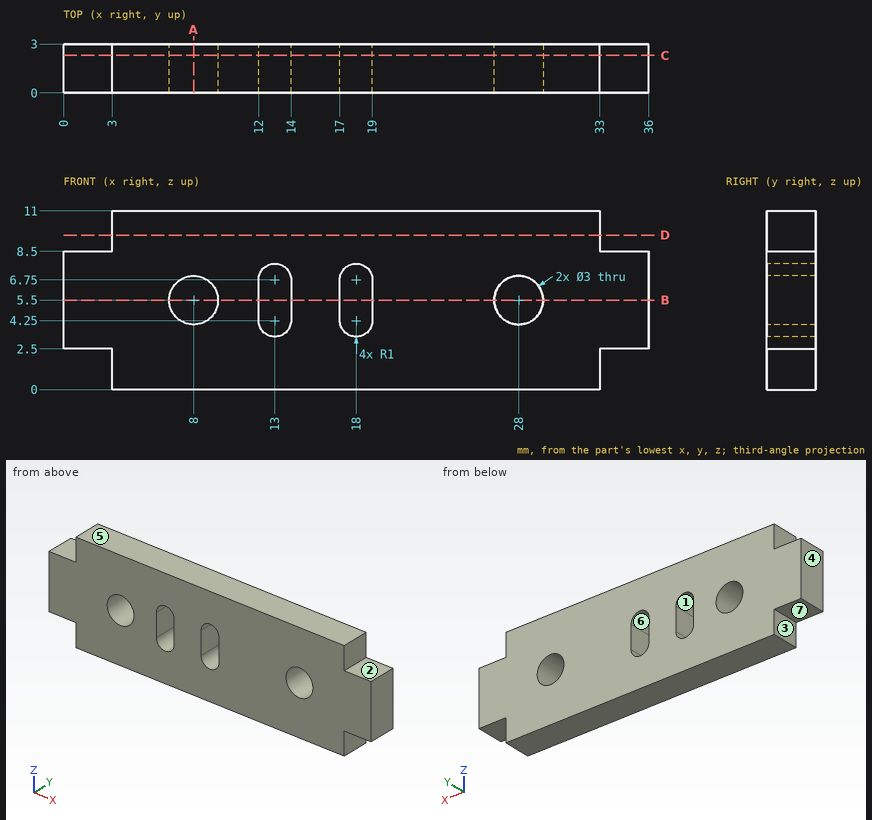
The drawing under review shows one solid part. Ordinate dimensions are in mm from its lowest x, y, z. A direction names the side the tool comes from. Round coordinates to 2 decimals unless told otherwise and drop trailing zeros. Write each loop counter-clockwise with the first axis right and the second up, starting at its lowest first coordinate (ties: lowest second). Pieces come first, ordered by that corner, then holes. Notation, with made-up numbers: (-1, 46) - (40, 46) arc R33 cw to (40, 75) - close; hole circle Ø3 at (5, 13.25). An arc over 180 degrees is marked (long way). Put each result on its own line as item: value.
Q1. We need section D-D (z = 9.5). Give the boundary of the cut face in (x, y), and give its area (3 significant figures).
Solved:
outline: (3, 0) - (33, 0) - (33, 3) - (3, 3) - close
area: 90.0 mm2
Q2. Wall thickness on probe 1 along Z at (x, y) = (28, 1.25); probe 2 along X at (y, z) = (2.7, 4.5); probe 3 along X at (y, z) = (2.8, 5): over which ranges is each line inside the solid? List them lowest first.
Solved:
probe 1: z = 0 to 4, 7 to 11
probe 2: x = 0 to 6.88, 9.12 to 12, 14 to 17, 19 to 26.88, 29.12 to 36
probe 3: x = 0 to 6.59, 9.41 to 12, 14 to 17, 19 to 26.59, 29.41 to 36
Q3. We need section B-B (z = 5.5). Give the boundary of the cut face in (x, y), and give its area (3 significant figures).
Solved:
outline: (0, 0) - (6.5, 0) - (6.5, 3) - (0, 3) - close; (9.5, 0) - (12, 0) - (12, 3) - (9.5, 3) - close; (14, 0) - (17, 0) - (17, 3) - (14, 3) - close; (19, 0) - (26.5, 0) - (26.5, 3) - (19, 3) - close; (29.5, 0) - (36, 0) - (36, 3) - (29.5, 3) - close
area: 78.0 mm2
Q4. Machinability: for the marked faces 1, 2 and 3, which of the approach directions +Z, -Z, +X, -X, +Y, -Y give a long, thin tool a straight path to every point of the face, cutting with its end or side? Answer none if there is none.
Solved:
face 1: +Y, -Y
face 2: +Z, +X, +Y, -Y
face 3: -Z, -X, +Y, -Y
Q5. Mouldability with a two-part tool opening along Z and no side actions: class the marked faces 4, 5, 6 and 7 as released by +Z, released by -Z, zero draft, split by the parting line, or undercut.
Solved:
face 4: zero draft
face 5: released by +Z
face 6: undercut
face 7: released by -Z
Q6. Insertion check: pin 1 Ø0.9 at (x, y) = (35, 1) entering from +Z; pin 2 Ø1.2 at (y, z) = (2, 9.5) entering from -X; pin 3 Ø1.5 at (x, y) = (2, 1) entering from -Z. Each pin has a flat end and moves straight along its axis. Give the tip position at first contact, or say it passes through.
Solved:
pin 1: stops at z = 8.5
pin 2: stops at x = 3
pin 3: stops at z = 2.5
Q7. We need section A-A (x = 8). Give the boundary of the cut face in (y, z), and give its area (3 significant figures).
Solved:
outline: (0, 0) - (3, 0) - (3, 4) - (0, 4) - close; (0, 7) - (3, 7) - (3, 11) - (0, 11) - close
area: 24.0 mm2
Q8. We need section C-C (y = 2.3). Give the boundary of the cut face in (x, z), and give its area (3 significant figures).
Solved:
outline: (0, 2.5) - (3, 2.5) - (3, 0) - (33, 0) - (33, 2.5) - (36, 2.5) - (36, 8.5) - (33, 8.5) - (33, 11) - (3, 11) - (3, 8.5) - (0, 8.5) - close; hole circle Ø3 at (8, 5.5); hole (12, 4.25) arc R1 ccw to (14, 4.25) - (14, 6.75) arc R1 ccw to (12, 6.75) - close; hole (17, 4.25) arc R1 ccw to (19, 4.25) - (19, 6.75) arc R1 ccw to (17, 6.75) - close; hole circle Ø3 at (28, 5.5)
area: 336 mm2
